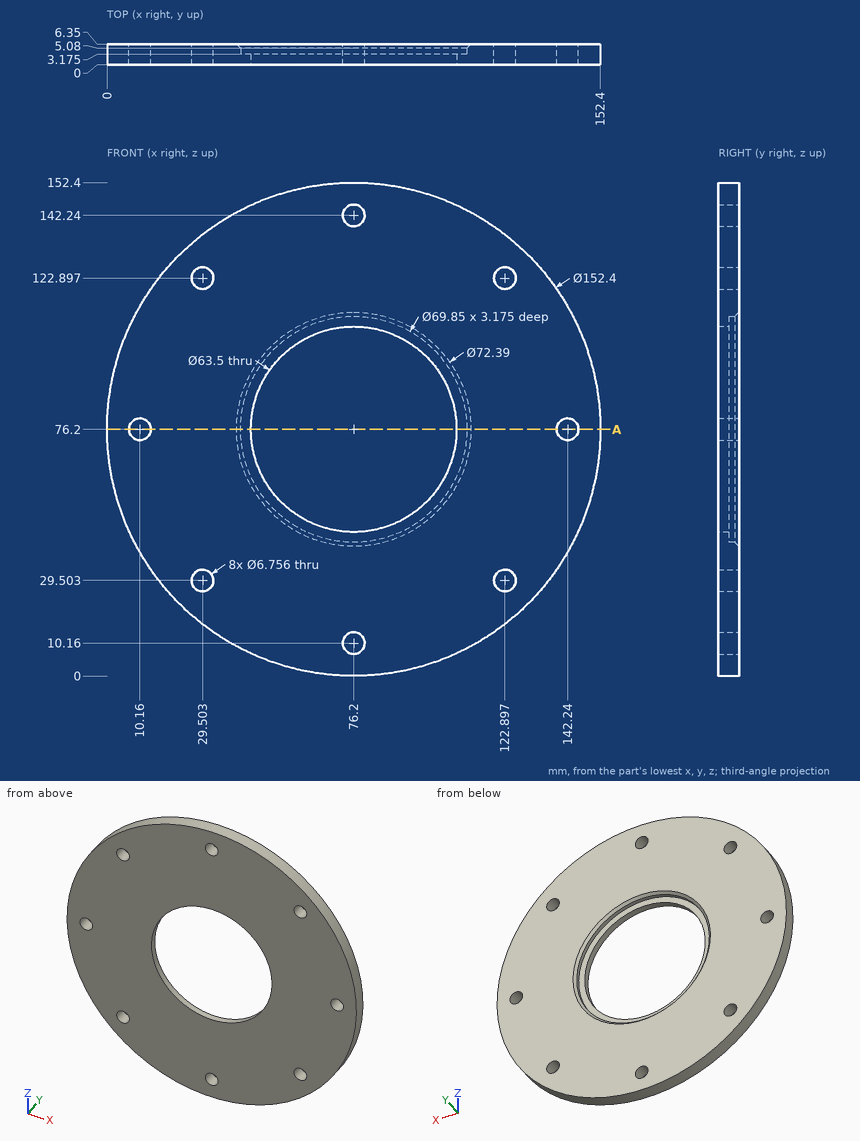
Input: dimensioned drawing with shaded views. Units: mm. Origin: part minimum x, y, z. Give positions to 0.01 mm unless a question says otherwise; leave off trailing zeros.
1. First-contact query: pin 1 (6 mm diameter, centred on x = 122.9, z = 29.5, fed in from -Y); pin 2 (3 mm diameter, centred on x = 68.5, y = 2.5, fed in from -Z); pin 3 (2 mm diameter, centred on x = 50.5, y = 5, fed in from -Z) (1 decimal); pin 4 (3 mm diameter, centred on y = 3, z = 62, fed in from +X). Flat tips, straight axial feed; report the tip coordinate or a pass-through.
2. Material intervals for line 1 along Y through (x, z) = (75, 111) (1 decimal); line 2 along Z through (x, y) = (72, 1) (1 decimal); line 3 along Z through (x, y) = (82.5, 5), sorted ascending.
3. Section query A-A (z = 76.2). Count the separate pieces of the cut face and the enclosed holes in it, then the cut area to 3 significant figures.
Output values:
1. pin 1: passes through
1. pin 2: stops at z = 0.25
1. pin 3: stops at z = 4.1
1. pin 4: stops at x = 151.33
2. line 1: y = 0 to 3.2
2. line 2: z = 0.1 to 44.7, 107.7 to 152.3
2. line 3: z = 0.26 to 41.85, 110.55 to 152.14
3. separate pieces: 4
3. enclosed holes: 0
3. area: 457 mm2
